```python
from build123d import *

# Parameters (mm, degrees)
F1_DEPTH      = 38.1
F1_DEPTH_BACK = 38.1
F2_R          = 5.08


with BuildPart() as f1:
    # F0 (on Front) → F1 (new body, two sides)
    with BuildSketch(Plane.XZ) as f1_sk:
        Polygon((-31.75, 69.85), (-31.75, -57.15), (-25.4, -57.15), (-25.4, 63.5), (12.7, 63.5), (12.7, -57.15), (19.05, -57.15), (19.05, 69.85), align=None)
    extrude(amount=F1_DEPTH)
    extrude(f1_sk.sketch, amount=-F1_DEPTH_BACK)

    # F2
    f2_edges = [f1.edges().sort_by_distance(p)[0] for p in [
        (-31.75, 0, 69.85),
        (19.05, 0, 69.85),
        (-25.4, 0, 63.5),
        (12.7, 0, 63.5),
    ]]
    fillet(f2_edges, radius=F2_R)


solid = f1.part
```
Geometry check sheet. Reference: the model listing, model coordinates, mm. A direction names the side the tool comes from. Coordinates: 2 decimals unless noted, no trailing zeros. Order: outer loops, then holes, each group sorted by start corner. A loop starts at its lowest first (then second) coordinate and runs counter-clockwise, first axis right, second up. Notation, with made-up numbers: (-32, 22.25) - (-9, 22.25) arc R16 ccw to (-9, 48.25) - close; hole circle Ø4 at (12.5, -16). An arc over 180 degrees is marked (long way). Answer as a JSON object with one key per item and string values. Group by question number.
Item 1: Sectioned sample at B-B, the plane y = -24.5. Record the cut outline in (x, z), and give its area (3 significant figures).
Item 2: Depth check by flat-ended pin: pin 1 Ø6 at (x, y) = (3, 0) entering from -Z. Enter the tip coordinate at first touch or a pass-through.
Item 3: Tool access check on faces 1 (the face through (-23.872, -0.533, 62.051)), 2 (the face through (-29, -1, -57.15)). Record the directions out of +Z, -Z, +X, -X, +Y, -Y that give a thin tool (end or side, any length) a straight path to the whole face; none if there is none.
Item 4: Sectioned sample at A-A, the plane z = -6.5. Record the cut outline in (x, y).
Item 5: Sectioned sample at C-C, the plane x = -1. Record the cut outline in (y, z).
Item 6: Scan lines: probe 1 along X at (y, z) = (-11.5, -27); probe 2 along Z at (x, y) = (-5, -6). Record each from-to range of solid material in increasing order.
Item 7: Draft check along X on faces 3 (the face through (-7, -1, 63.5)), 4 (the face through (14, 38.1, 16)), 5 (the face through (-31.75, -1, 5)), 6 (the face through (19.05, -1, 3)). Enter one of: +X half, -X half, draft (parallel to the pull), parting line (faces both ways), or undercut.
Resolved:
{
 "1": {"outline": "(-31.75, -57.15) - (-25.4, -57.15) - (-25.4, 58.42) arc R5.08 cw to (-20.32, 63.5) - (7.62, 63.5) arc R5.08 cw to (12.7, 58.42) - (12.7, -57.15) - (19.05, -57.15) - (19.05, 64.77) arc R5.08 ccw to (13.97, 69.85) - (-26.67, 69.85) arc R5.08 ccw to (-31.75, 64.77) - close", "area": "1,850 mm^2"},
 "2": {"pin 1": "z = 63.5"},
 "3": {"face 1": "-Z, +Y, -Y", "face 2": "-Z, +X, -X, +Y, -Y"},
 "4": {"outline": "(-31.75, -38.1) - (-25.4, -38.1) - (-25.4, 38.1) - (-31.75, 38.1) - close; (12.7, -38.1) - (19.05, -38.1) - (19.05, 38.1) - (12.7, 38.1) - close"},
 "5": {"outline": "(-38.1, 63.5) - (38.1, 63.5) - (38.1, 69.85) - (-38.1, 69.85) - close"},
 "6": {"probe 1": "-31.75 to -25.4, 12.7 to 19.05", "probe 2": "63.5 to 69.85"},
 "7": {"face 3": "undercut", "face 4": "draft", "face 5": "-X half", "face 6": "+X half"}
}
